Could you check a few things on this model? Use its own coordinates, in mm. Face numbers are marked on the shaded views. A direction names the side the tool comes from. Coordinates: 2 decimals unless noted, no trailing zeros. Loops run counter-clockwise (first coordinate to the right, second up) from the corner with the lowest first, then second, coordinate; pieces in that order, holes last. Notation, with made-up numbers: (-36, 61.5) - (-25, 61.5) arc R19 ccw to (-25, 82.5) - close; hole circle Ø6 at (20, -20.75). An arc over 180 degrees is marked (long way). One line per question, with ' | ' between items. Start each with the question number.
1. Please list where these lines run through material, in increasing order: L1, parallel to X at y = 15, z = -35; L2, parallel to Z at x = 5, y = 26; L3, parallel to Y at x = -23, z = -87. Write a range as [from, to].
2. I'm going to push flat-ended pins straight in: P1, Ø8, axis at y = 21.5, z = -40, coming from the +X side; P2, Ø5.5, axis at x = 28.5, y = -6, coming from the -Z side; P3, Ø10, axis at x = -5.5, y = 21.5, coming from the +Z side; P4, Ø6, axis at y = 25, z = -87.5, coming from the +X side. Where does each tip first touch, or does it pass through?
3. We'd pull the mould along X, two halves only. Please class the marked faces 1, 2 and 3: pulls with the +X half, pulls with the -X half, needs draft (parallel to the pull), parting line crosses it, or undercut.
4. Which directions (+Z, -Z, +X, -X, +Y, -Y) give clear straight access to the entire face, cutting with the end or side of a thin tool? Please do the marked faces 4 and 5.
5. I want a section at A-A, the plane x = 0. Write out the boundary of the cut face in (y, z).
6. I want a section at D-D, the plane z = -37. Write out the boundary of the cut face in (x, y), then the cut area to 3 significant figures.
7. I want a section at B-B, the plane y = 25. Write out the boundary of the cut face in (x, z), then the cut area to 3 significant figures.
8. I want a section at C-C, the plane z = -87.5. Write out the boundary of the cut face in (x, y), then the cut area to 3 significant figures.
from build123d import *

# Parameters (mm, degrees)
F0_R      = 7.5
F0_R_2    = 5
F1_DEPTH  = 2.5
F2_DEPTH  = 7
F3_R      = 5
F4_DEPTH  = 2
F5_DEPTH  = 90
F7_DEPTH  = 3
F6_R      = 5
F8_DEPTH  = 3
F10_DEPTH = 3
F9_R      = 5
F11_DEPTH = 3
F12_R     = 10
F13_R     = 5
F14_R     = 5


with BuildPart() as f1:
    # F0 (on Top) → F1 (new body)
    with BuildSketch(Plane.XY):
        Circle(F0_R)
        Circle(F0_R_2, mode=Mode.SUBTRACT)
    extrude(amount=-F1_DEPTH)

    # F0 (on Top) → F2 (join)
    with BuildSketch(Plane.XY):
        Circle(F0_R_2)
    extrude(amount=-F2_DEPTH)

    # F3 (on face) → F4 (join)
    with BuildSketch(Plane(origin=(0, 0, -7), x_dir=(1, 0, 0), z_dir=(0, 0, -1))):
        with BuildLine():
            Line((22, 16.5828760482), (25, 16.5831239518))
            ThreePointArc((25, 16.5831239518), (0, 30), (-25, 16.5831239518))
            Line((-25, 16.5831239518), (-22, 16.5828760482))
            Line((-22, 16.5828760482), (-22, 0))
            Line((-22, 0), (-22, -16.5831239518))
            Line((-22, -16.5831239518), (-25, -16.5831239518))
            ThreePointArc((-25, -16.5831239518), (0, -30), (25, -16.5831239518))
            Line((25, -16.5831239518), (22, -16.5831239518))
            Line((22, -16.5831239518), (22, 0))
            Line((22, 0), (22, 16.5828760482))
        make_face()
        Circle(F3_R, mode=Mode.SUBTRACT)
        Circle(F3_R)
    extrude(amount=F4_DEPTH)

    # F3 (on face) → F4, piece 2 (join)
    with BuildSketch(Plane(origin=(0, 0, -7), x_dir=(1, 0, 0), z_dir=(0, 0, -1))):
        with BuildLine():
            Line((-25, 0), (-25, 16.5831239518))
            ThreePointArc((-25, 16.5831239518), (-30, 0), (-25, -16.5831239518))
            Line((-25, -16.5831239518), (-25, 0))
        make_face()
    extrude(amount=F4_DEPTH)

    # F3 (on face) → F4, piece 3 (join)
    with BuildSketch(Plane(origin=(0, 0, -7), x_dir=(1, 0, 0), z_dir=(0, 0, -1))):
        with BuildLine():
            ThreePointArc((25, -16.5831239518), (28.7228132327, -8.6602540378), (30, 0))
            ThreePointArc((30, 0), (28.7228132327, 8.6602540378), (25, 16.5831239518))
            Line((25, 16.5831239518), (25, 0))
            Line((25, 0), (25, -16.5831239518))
        make_face()
    extrude(amount=F4_DEPTH)

    # F3 (on face) → F5 (join)
    with BuildSketch(Plane(origin=(0, 0, -7), x_dir=(1, 0, 0), z_dir=(0, 0, -1))):
        Polygon((-22, 16.5828760482), (-25, 16.5831239518), (-25, 0), (-25, -16.5831239518), (-22, -16.5831239518), (-22, 0), align=None)
        Polygon((25, 0), (25, 16.5831239518), (22, 16.5828760482), (22, 0), (22, -16.5831239518), (25, -16.5831239518), align=None)
    extrude(amount=F5_DEPTH)

    # F6 (on face) → F7 (cut)
    with BuildSketch(Plane.YZ.offset(25)):
        Polygon((16.5831239518, -97), (-16.5831239518, -9), (-16.5831239518, -97), align=None)
    extrude(amount=-F7_DEPTH, mode=Mode.SUBTRACT)

    # F6 (on face) → F8 (join)
    with BuildSketch(Plane.YZ.offset(25)):
        Polygon((16.5831239518, -9), (16.5831239518, -97), (46.5831239518, -97), align=None)
        with Locations((25, -87.5)):
            Circle(F6_R, mode=Mode.SUBTRACT)
    extrude(amount=-F8_DEPTH)

    # F9 (on face) → F10 (cut)
    with BuildSketch(Plane(origin=(-25, 0, 0), x_dir=(0, -1, 0), z_dir=(-1, 0, 0))):
        Polygon((16.5831239518, -97), (16.5831239518, -9), (-16.5831239518, -97), align=None)
    extrude(amount=-F10_DEPTH, mode=Mode.SUBTRACT)

    # F9 (on face) → F11 (join)
    with BuildSketch(Plane(origin=(-25, 0, 0), x_dir=(0, -1, 0), z_dir=(-1, 0, 0))):
        Polygon((-46.5831239518, -97), (-16.5831239518, -97), (-16.5831239518, -9), align=None)
        with Locations((-25, -87.5)):
            Circle(F9_R, mode=Mode.SUBTRACT)
    extrude(amount=-F11_DEPTH)

    # F12
    f12_edges = [f1.edges().sort_by_distance(p)[0] for p in [
        (-23.5, 46.583124, -97),
        (23.5, 46.583124, -97),
    ]]
    fillet(f12_edges, radius=F12_R)

    # F13
    f13_edges = [f1.edges().sort_by_distance(p)[0] for p in [
        (-23.5, 16.583124, -97),
    ]]
    fillet(f13_edges, radius=F13_R)

    # F14
    f14_edges = [f1.edges().sort_by_distance(p)[0] for p in [
        (23.5, 16.583124, -97),
    ]]
    fillet(f14_edges, radius=F14_R)


solid = f1.part
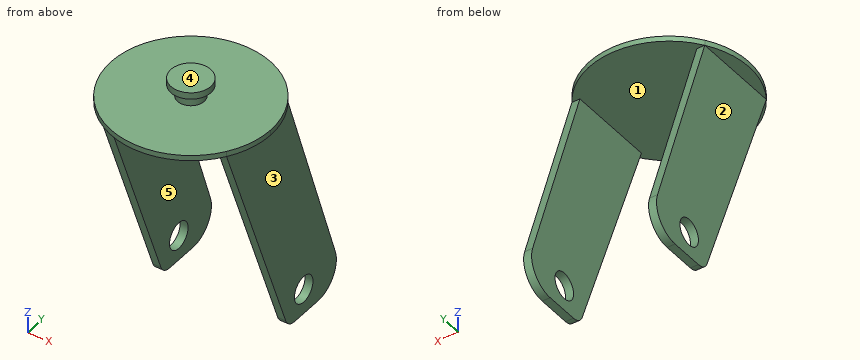
Results are:
1) L1: x = [-25, -22], [22, 25] | L2: z = [-9, -7] | L3: y = [12.81, 20.03], [29.97, 42.61]
2) P1: stops at x = 25 | P2: stops at z = -9 | P3: stops at z = -7 | P4: passes through
3) face 1: undercut | face 2: pulls with the -X half | face 3: pulls with the +X half
4) face 4: +Z, +X, -X, +Y, -Y | face 5: -Z, +Y, -Y
5) outline: (-30, -9) - (30, -9) - (30, -7) - (5, -7) - (5, -2.5) - (7.5, -2.5) - (7.5, 0) - (-7.5, 0) - (-7.5, -2.5) - (-5, -2.5) - (-5, -7) - (-30, -7) - close
6) outline: (-25, -6.03) - (-22, -6.03) - (-22, 26.13) - (-25, 26.13) - close; (22, -6.03) - (25, -6.03) - (25, 26.13) - (22, 26.13) - close | area: 193 mm2
7) outline: (-25, -97) - (-22, -97) - (-22, -92.5) - (-25, -92.5) - close; (-25, -82.5) - (-22, -82.5) - (-22, -33.69) - (-25, -33.69) - close; (-16.58, -9) - (16.58, -9) - (16.58, -7) - (-16.58, -7) - close; (22, -97) - (25, -97) - (25, -92.5) - (22, -92.5) - close; (22, -82.5) - (25, -82.5) - (25, -33.69) - (22, -33.69) - close | area: 386 mm2
8) outline: (-25, 13) - (-22, 13) - (-22, 20) - (-25, 20) - close; (-25, 30) - (-22, 30) - (-22, 42.6) - (-25, 42.6) - close; (22, 13) - (25, 13) - (25, 20) - (22, 20) - close; (22, 30) - (25, 30) - (25, 42.6) - (22, 42.6) - close | area: 118 mm2
